Autodesk Inventor part; units mm, degrees
ref_plane "Work Plane1" through (1.525, 0, 0) normal (0, 0, 1) x (1, 0, 0)
ref_plane "YZ Plane" through (0, 0, 0) normal (1, 0, 0) x (0, 1, 0)
ref_plane "XZ Plane" through (0, 0, 0) normal (0, 1, 0) x (-1, 0, 0)
sketch "Sketch1" plane through (0, 0, 0) normal (0, 0, 1) x (1, 0, 0)
  line L0 (0, 5.815) -> (0, 4)
  line L1 (3, 4) -> (16, 4)
  line L2 (16, 4) -> (16, 0)
  line L3 (16, 0) -> (-0.6001, 0)
  line L4 (-3.9201, 0) -> (19.32, 0)
  line L5 (-0.6001, 0) -> (-0.6001, 5.815)
  line L6 (-0.6001, 5.815) -> (0, 5.815)
  line L7 (3, 4) -> (2.3865, 4)
  line L8 (2.3865, 4) -> (0, 4)
  line L9 (0, -1.163) -> (0, 6.978)
  dimension "d0" = 16
  dimension "d1" = 13
  dimension "d2" = 8
  dimension "d9" = 0.6001
  dimension "d10" = 11.63
  dimension "d13" = 0.6136
  dimension "d14" = 8
revolve "Body" add sketch "Sketch1" angle 360 about axis through (16, 0, 0) along (-1, 0, 0)
sketch "Sketch2" plane through (-0.6001, 0, 0) normal (-1, 0, 0) x (0, 0, 1)
  line L0 (0, 7.5056) -> (6.5, 3.7528)
  line L1 (6.5, 3.7528) -> (6.5, -3.7528)
  line L2 (6.5, -3.7528) -> (0, -7.5056)
  line L3 (0, -7.5056) -> (-6.5, -3.7528)
  line L4 (-6.5, -3.7528) -> (-6.5, 3.7528)
  line L5 (-6.5, 3.7528) -> (0, 7.5056)
  point P0 (0, 0)
  point P1 (0, 0)
  dimension "d11" = 13
extrude "Head" add sketch "Sketch2" along normal blind 4.7
sketch "Sketch4" plane through (0, 0, 0) normal (0, 0, 1) x (1, 0, 0)
  line L0 (-5.3001, 6.5) -> (-5.3001, 7.5056)
  line L1 (-5.3001, 7.5056) -> (-4.7195, 7.5056)
  line L2 (-4.7195, 7.5056) -> (-5.3001, 6.5)
  line L3 (-6.2401, 0) -> (0.3399, 0)
  line L4 (-0.6001, 7.5056) -> (-5.3001, 7.5056)
  line L5 (-5.3001, 3.7528) -> (-5.3001, 7.5056)
  dimension "d5" = 30
  dimension "d19" = 13
revolve "Chamfer1" cut sketch "Sketch4" angle 360 about axis through (-10, 0, 0) along (1, 0, 0)
thread "Thread"
chamfer "Chamfer2" distance 0.6134 distance2 0.6136 1 edges at (16, -4, 0) measured on face at (16, -0.6859, -0.8072)
ref_plane "Work Plane1" through (1.525, 0, 0) normal (0, 0, 1) x (1, 0, 0)
equation "\"d0\" = NLG"
equation "\"d1\" = GEL"
equation "\"d2\" = GD"
equation "\"d10\" = SD2"
equation "\"d14\" = BDM"
equation "\"d11\" = SW"
equation "\"d3\" = KOH - SD"
equation "\"d5\" = ANG1"
equation "\"d19\" = SW0"
equation "\"d15\" = GEL"
equation "\"d6\" = -0.5 * SPD + 0.5 * GD"
equation "\"NLG\" = 16"
equation "\"GD\" = NND"
equation "\"BDM\" = NND"
equation "\"KOH\" = 5.3"
equation "\"GEL\" = 13"
equation "\"SW\" = 13"
equation "\"SW0\" = 13"
equation "\"SPD\" = NND - 1.2269 * PTC"
equation "\"SD2\" = 11.63"
equation "\"SD\" = 0.6"
equation "\"ANG1\" = 30deg"
equation "\"GAL\" = 0.61345 * PTC"
equation "\"GUL\" = 0.61345 * PTC"
equation "\"RR\" = 0.4"
equation "\"GD1\" = THREADDIA - 1.2269 * PTC"
equation "\"THREADDIA\" = 8"
equation "\"SDH\" = SD2"
equation "\"TOA\" = 30deg"
equation "\"PTC\" = 1"
equation "\"NND\" = 8"
equation "\"E0\" = 1.155 * SW"
properties part number "ISO 8676 - M8 x 1 x 16(3)" material "Stainless Steel, 440C"
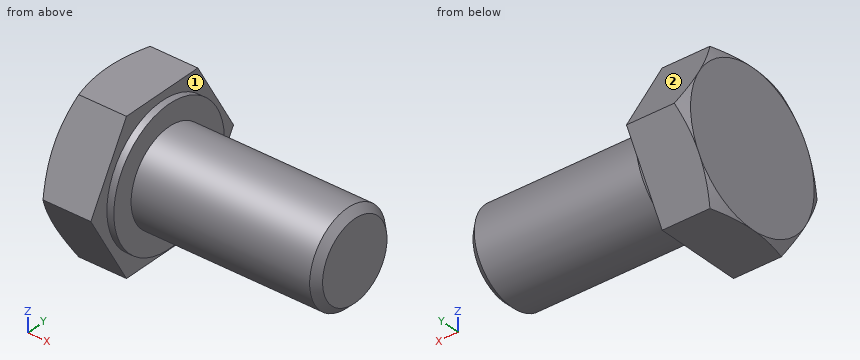
Read the model definition and answer for the solid it produces. Units are mm, in the model's axes. Face numbers are marked on the shaded views. A direction names the side the tool comes from. Give positions to 0.01 mm unless a question says otherwise; leave off trailing zeros. Loops run counter-clockwise (first coordinate to the right, second up) from the corner with the lowest first, then second, coordinate; pieces in that order, holes last.
Item 1: The part is cut by section A-A (x = -1). Write down the section's boundary in (y, z), and give its area (3 significant figures).
Item 2: Each of these flat-tipped pins is pushed along its axis until it touches: pin 1 Ø4 at (x, y) = (8.5, -2.5) entering from -Z; pin 2 Ø1.5 at (x, z) = (-2.5, 2) entering from -Y; pin 3 Ø6 at (x, y) = (7.5, -1.5) entering from +Z. Where does it stop, or does it pass through?
Item 3: For the marked faces 1 and 2, determine the directions among +Z, -Z, +X, -X, +Y, -Y from which every point of the face is accessible in a straight line to the end or side of a thin tool.
Item 4: Find the intervals of material crossed by line 1 along X through (y, z) = (-4.75, 3); line 2 along X through (y, z) = (5.5, -2.5); line 3 along Y through (x, z) = (2.75, -1.25), in increasing order.
Item 5: The part is cut by section B-B (x = 2.5). Write down the section's boundary in (y, z), and give its area (3 significant figures).
Taken from the geometry:
1. outline: (-7.51, 0) - (-3.75, -6.5) - (3.75, -6.5) - (7.51, 0) - (3.75, 6.5) - (-3.75, 6.5) - close
1. area: 146 mm2
2. pin 1: stops at z = -3.97
2. pin 2: stops at y = -6.78
2. pin 3: stops at z = 4
3. face 1: +X
3. face 2: +Z, +X, -X, +Y
4. line 1: x = -5.3 to 0
4. line 2: x = -5.3 to -0.6
4. line 3: y = -3.8 to 3.8
5. outline: circle Ø8 at (0, 0)
5. area: 50.3 mm2
